```python
from build123d import *

# Parameters (mm, degrees)
SKETCH1_R                                     = 53.086
SKETCH1_R_2                                   = 12.7
BOSS_EXTRUDE1_DEPTH                           = 12.7
F_1_4_20_TAPPED_HOLE1_AT_2_COUNT              = 2
F_1_4_20_TAPPED_HOLE1_AT_2_PITCH              = 50.8
F_1_4_20_TAPPED_HOLE1_AT_3_COUNT              = 2
F_1_4_20_TAPPED_HOLE1_AT_3_PITCH              = 71.842048969
F_1_4_20_TAPPED_HOLE1_AT_4_COUNT              = 2
F_1_4_20_TAPPED_HOLE1_AT_4_PITCH              = 50.8
CBORE_FOR_1_4_BUTTON_HEAD_CAP_SCREW1_AT_COUNT = 2
CBORE_FOR_1_4_BUTTON_HEAD_CAP_SCREW1_AT_PITCH = 35.921024484
CBORE_FOR_1_4_BUTTON_HEAD_CAP_SCREW1_2_COUNT  = 2
CBORE_FOR_1_4_BUTTON_HEAD_CAP_SCREW1_2_PITCH  = 50.8
CBORE_FOR_1_4_BUTTON_HEAD_CAP_SCREW1_3_COUNT  = 2
CBORE_FOR_1_4_BUTTON_HEAD_CAP_SCREW1_3_PITCH  = 35.921024484
CHAMFER1_SIZE                                 = 0.254


with BuildPart() as part:
    # Sketch1 → Boss-Extrude1 (new body)
    with BuildSketch(Plane(origin=(0, 0, 0), x_dir=(1, 0, 0), z_dir=(0, 1, 0))):
        Circle(SKETCH1_R)
        Circle(SKETCH1_R_2, mode=Mode.SUBTRACT)
    extrude(amount=-BOSS_EXTRUDE1_DEPTH)

    # Sketch4 → 1/4-20 Tapped Hole1 (revolve, cut)
    with BuildSketch(Plane(origin=(0, 0, 35.921024484), x_dir=(0, 0, 1), z_dir=(1, 0, 0))):
        Polygon((0, 0), (0, 12.7), (3.81, 12.7), (2.5527, 11.4427), (2.5527, 1.2573), (3.81, 0), align=None)
    f_1_4_20_tapped_hole1 = revolve(axis=Axis((0, 6.35, 35.921024484), (0, -1, 0)), mode=Mode.SUBTRACT)

    # 1/4-20 Tapped Hole1 at 2: 1/4-20 Tapped Hole1 ×2
    with Locations(*[Vector(-0.707106781, 0, -0.707106781) * (i * F_1_4_20_TAPPED_HOLE1_AT_2_PITCH) for i in range(1, F_1_4_20_TAPPED_HOLE1_AT_2_COUNT)]):
        add(f_1_4_20_tapped_hole1, mode=Mode.SUBTRACT)

    # 1/4-20 Tapped Hole1 at 3: 1/4-20 Tapped Hole1 ×2
    with Locations(*[(0, 0, -i * F_1_4_20_TAPPED_HOLE1_AT_3_PITCH) for i in range(1, F_1_4_20_TAPPED_HOLE1_AT_3_COUNT)]):
        add(f_1_4_20_tapped_hole1, mode=Mode.SUBTRACT)

    # 1/4-20 Tapped Hole1 at 4: 1/4-20 Tapped Hole1 ×2
    with Locations(*[Vector(0.707106781, 0, -0.707106781) * (i * F_1_4_20_TAPPED_HOLE1_AT_4_PITCH) for i in range(1, F_1_4_20_TAPPED_HOLE1_AT_4_COUNT)]):
        add(f_1_4_20_tapped_hole1, mode=Mode.SUBTRACT)

    # Sketch5 → CBORE for 1/4 Button Head Cap Screw1 (revolve, cut)
    with BuildSketch(Plane(origin=(-17.960512242, 0, 17.960512242), x_dir=(0, 0, 1), z_dir=(1, 0, 0))):
        Polygon((0, 0), (0, 12.7), (3.8989, 12.7), (3.2639, 12.065), (3.2639, 6.7564), (5.95376, 6.7564), (5.95376, 0.635), (6.58876, 0), align=None)
    cbore_for_1_4_button_head_cap_screw1 = revolve(axis=Axis((-17.960512242, 6.35, 17.960512242), (0, -1, 0)), mode=Mode.SUBTRACT)

    # CBORE for 1/4 Button Head Cap Screw1 at: CBORE for 1/4 Button Head Cap Screw1 ×2
    with Locations(*[(0, 0, -i * CBORE_FOR_1_4_BUTTON_HEAD_CAP_SCREW1_AT_PITCH) for i in range(1, CBORE_FOR_1_4_BUTTON_HEAD_CAP_SCREW1_AT_COUNT)]):
        add(cbore_for_1_4_button_head_cap_screw1, mode=Mode.SUBTRACT)

    # CBORE for 1_4 Button Head Cap Screw1 2: CBORE for 1/4 Button Head Cap Screw1 ×2
    with Locations(*[Vector(0.707106781, 0, -0.707106781) * (i * CBORE_FOR_1_4_BUTTON_HEAD_CAP_SCREW1_2_PITCH) for i in range(1, CBORE_FOR_1_4_BUTTON_HEAD_CAP_SCREW1_2_COUNT)]):
        add(cbore_for_1_4_button_head_cap_screw1, mode=Mode.SUBTRACT)

    # CBORE for 1_4 Button Head Cap Screw1 3: CBORE for 1/4 Button Head Cap Screw1 ×2
    with Locations(*[(i * CBORE_FOR_1_4_BUTTON_HEAD_CAP_SCREW1_3_PITCH, 0, 0) for i in range(1, CBORE_FOR_1_4_BUTTON_HEAD_CAP_SCREW1_3_COUNT)]):
        add(cbore_for_1_4_button_head_cap_screw1, mode=Mode.SUBTRACT)

    # Chamfer1
    chamfer1_edges = [part.edges().sort_by_distance(p)[0] for p in [
        (-53.086, 0, 0),
        (-53.086, -12.7, 0),
        (-12.7, -12.7, 0),
        (-12.7, 0, 0),
    ]]
    chamfer(chamfer1_edges, length=CHAMFER1_SIZE)


solid = part.part
```
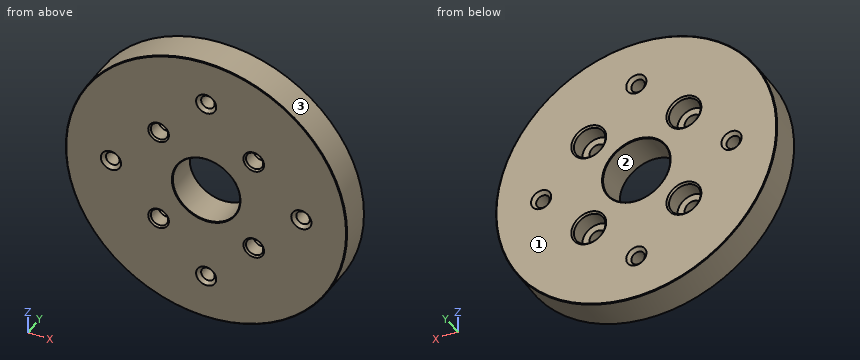
Check sheet for the modelled part. Datum: model origin and axes. Units: mm. Face numbers are marked on the shaded views. Give positions to 0.01 mm unless a question says otherwise; leave off trailing zeros. Answer as a JSON object with one key per item and string values. Group by question number.
1) Sectioned sample at A-A (x = 0). Give the number of separate pieces and of enclosed holes in the cut face, then the cut area to 3 significant figures.
2) Release check for a two-part mould opening along Z. For the marked faces 1, 2 and 3 record: pulls with the +Z half, pulls with the -Z half, needs draft (parallel to the pull), parting line crosses it, or undercut.
3) Depth check by flat-ended pin: P1, Ø2, axis at x = -14, y = -5.5, coming from the -Z side; P2, Ø1, axis at y = -4, z = -9.5, coming from the -X side; P3, Ø7.5, axis at x = -17.96, z = -17.96, coming from the -Y side. Enter the tip coordinate at first touch or a pass-through.
4) Thickness scan on probe 1 along Z at (x, y) = (-18.5, -3.5); probe 2 along X at (y, z) = (-8.5, 0); probe 3 along X at (y, z) = (-8, -16.5). Record the ranges inside material, lowest first. Write a range as from..to.
Geometry results:
{
 "1": {"separate pieces": "4", "enclosed holes": "0", "area": "890 mm^2"},
 "2": {"face 1": "needs draft", "face 2": "undercut", "face 3": "parting line crosses it"},
 "3": {"P1": "stops at z = -51.47", "P2": "stops at x = -52.32", "P3": "stops at y = -12.55"},
 "4": {"probe 1": "z = -49.76..-23.89, -12.03..12.03, 23.89..49.76", "probe 2": "x = -53.09..-38.47, -33.37..-12.7, 12.7..33.37, 38.47..53.09", "probe 3": "x = -50.46..-20.88, -15.04..15.04, 20.88..50.46"}
}
